```python
from build123d import *

# Parameters (mm, degrees)
F0_W     = 107.845894
F0_H     = 62.084262
F1_DEPTH = 52.578
F2_R     = 18.151489
F3_DEPTH = 49.784
F4_R     = 17.028329
F5_DEPTH = 25.4


with BuildPart() as f1:
    # F0 (on Top) → F1 (new body)
    with BuildSketch(Plane.XY):
        Rectangle(F0_W, F0_H)
    extrude(amount=F1_DEPTH)

    # F2 (on face) → F3 (cut)
    with BuildSketch(Plane.XY.offset(52.578)):
        with Locations((-31.67621, 0)):
            Circle(F2_R)
    extrude(amount=-F3_DEPTH, mode=Mode.SUBTRACT)

    # F4 (on face) → F5 (cut)
    with BuildSketch(Plane.XY.offset(52.578)):
        with Locations((28.308643, 11.2424)):
            Circle(F4_R)
    extrude(amount=-F5_DEPTH, mode=Mode.SUBTRACT)


solid = f1.part
```
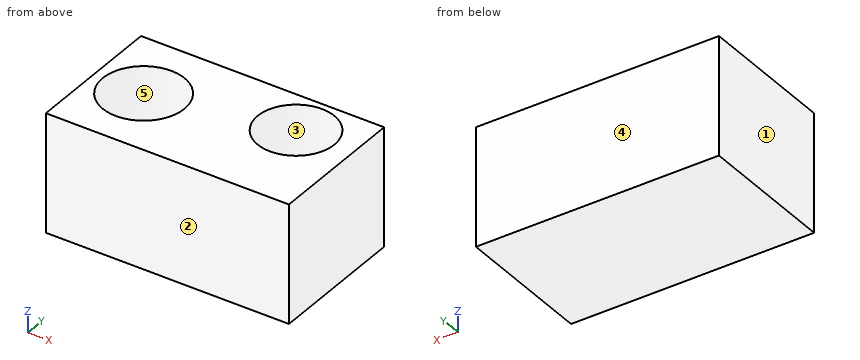
Read the model definition and answer for the solid it produces. Units are mm, in the model's axes. Face numbers are marked on the shaded views. A direction names the side the tool comes from. Give positions to 0.01 mm unless a question says otherwise; leave off trailing zeros. Write each loop counter-clockwise with the first axis right and the second up, starting at its lowest first coordinate (ties: lowest second). Pieces come first, ordered by that corner, then holes. Notation, with made-up numbers: M 87.5,-21 L 101.5,-21 A34 cw 101.5,13 Z; hole C 52.5,63.5 d2. An arc over 180 degrees is marked long. Put each result on its own line as item: value. Start each with the question number.
1. The part is cut by section C-C, the plane x = 23. Give the vertices of the cut face in (y, z).
2. The part is cut by section D-D, the plane z = 37. Give the vertices of the cut face in (x, y), and give its area (3 significant figures).
3. Consider line 1 along X through (y, z) = (10, 18.5); line 2 along X through (y, z) = (9, 3); line 3 along Z through (x, y) = (14.5, 7.5). Determine where each line is inside the solid, lowest interval first.
4. For a pull along Y with two mould halves and no side action, classify the marked faces 1, 2 and 3 as released by +Y, released by -Y, zero draft, split by the parting line, or undercut.
5. Which of the six approach directions +Z, -Z, +X, -X, +Y, -Y give full straight-line access (tool end or side, diameter ignored) to the marked faces 4 and 5?
6. The part is cut by section A-A, the plane z = 16. Give the vertices of the cut face in (x, y).
7. The part is cut by section B-B, the plane y = 0. Give the vertices of the cut face in (x, z).
8. This flat-tipped pin is pushed along its axis until it touches: pin 1 Ø8 at (x, y) = (39, 15.5) entering from +Z. Where does it stop, or does it pass through?
Final values:
1. outline: M -31.04,0 L 31.04,0 L 31.04,52.58 L 27.42,52.58 L 27.42,27.18 L -4.94,27.18 L -4.94,52.58 L -31.04,52.58 Z
2. outline: M -53.92,-31.04 L 53.92,-31.04 L 53.92,31.04 L -53.92,31.04 Z; hole C -31.68,0 d36.3; hole C 28.31,11.24 d34.06
2. area: 4,750 mm²
3. line 1: x = -53.92 to -46.82, -16.53 to 53.92
3. line 2: x = -53.92 to -47.44, -15.91 to 53.92
3. line 3: z = 0 to 27.18
4. face 1: zero draft
4. face 2: released by -Y
4. face 3: undercut
5. face 4: +Z, -Z, +X, -X, +Y
5. face 5: +Z
6. outline: M -53.92,-31.04 L 53.92,-31.04 L 53.92,31.04 L -53.92,31.04 Z; hole C -31.68,0 d36.3
7. outline: M -53.92,0 L 53.92,0 L 53.92,52.58 L 41.1,52.58 L 41.1,27.18 L 15.52,27.18 L 15.52,52.58 L -13.52,52.58 L -13.52,2.79 L -49.83,2.79 L -49.83,52.58 L -53.92,52.58 Z
8. pin 1: stops at z = 27.18
